Autodesk Inventor part; units mm, degrees
ref_plane "YZ Plane" through (0, 0, 0) normal (1, 0, 0) x (0, 1, 0)
ref_plane "XZ Plane" through (0, 0, 0) normal (0, 1, 0) x (-1, 0, 0)
ref_plane "XY Plane" through (0, 0, 0) normal (0, 0, 1) x (1, 0, 0)
sketch "Эскиз1" plane through (0, 0, 0) normal (0, 0, 1) x (1, 0, 0)
  line L0 (-4.6809, -0.7904) -> (-4.6809, 1.2096)
  line L1 (-4.6809, -13.7904) -> (-4.6809, -11.7904)
  line L2 (-4.6809, 1.2096) -> (-9.1809, 1.2096)
  line L3 (-10.1809, 0.2096) -> (-10.1809, -12.7904)
  line L4 (-9.1809, -13.7904) -> (-4.6809, -13.7904)
  arc A0 (-10.1809, -12.7904) -> (-9.1809, -13.7904) centre (-9.1809, -12.7904) ccw
  arc A1 (-9.1809, 1.2096) -> (-10.1809, 0.2096) centre (-9.1809, 0.2096) ccw
  line L5 (22.8191, -1.7904) -> (22.8191, -10.7904)
  line L6 (21.8191, -11.7904) -> (-4.6809, -11.7904)
  line L7 (-4.6809, -0.7904) -> (21.8191, -0.7904)
  arc A2 (22.8191, -1.7904) -> (21.8191, -0.7904) centre (21.8191, -1.7904) ccw
  arc A3 (21.8191, -11.7904) -> (22.8191, -10.7904) centre (21.8191, -10.7904) ccw
  arc A4 (-0.4309, -4.5404) -> (-0.4309, -8.0404) centre (-0.4309, -6.2904) ccw
  arc A5 (1.5691, -8.0404) -> (1.5691, -4.5404) centre (1.5691, -6.2904) ccw
  line L8 (-0.4309, -4.5404) -> (1.5691, -4.5404)
  line L9 (-0.4309, -8.0404) -> (1.5691, -8.0404)
  circle A6 centre (18.0691, -6.2904) radius 1.75
  point P0 (0, 0)
  point P1 (-10.1809, 1.2096)
  point P2 (-10.1809, -13.7904)
  point P3 (22.8191, -0.7904)
  point P4 (22.8191, -11.7904)
extrude "Выдавливание2" add sketch "Эскиз1" along normal blind 2
properties part number "Крепеж"
Here's how the part is built. I have some questions about the finished solid (model axes, mm). A direction names the side the tool comes from. Coordinates: 2 decimals unless noted, no trailing zeros. Order: outer loops, then holes, each group sorted by start corner. A loop starts at its lowest first (then second) coordinate and runs counter-clockwise, first axis right, second up.
Item 1: Which directions (+Z, -Z, +X, -X, +Y, -Y) give clear straight access to the entire face, cutting with the end or side of a thin tool? Please do faces 1 (the face through (6, -6, 0)), 2 (the face through (9, -11.79, 1)), 3 (the face through (-4.681, 0, 1)), 4 (the face through (1, -8.04, 1)), 5 (the face through (-9.88, -13.505, 0.986)).
Response values:
face 1: -Z, +X, -X, +Y, -Y
face 2: +Z, -Z, +X, -Y
face 3: +Z, -Z, +X, +Y
face 4: +Z, -Z
face 5: +Z, -Z, -X, -Y
Item 2: I'm going to push flat-ended pins straight in: pin 1 Ø1 at (y, z) = (0.5, 1.5) entering from +X; pin 2 Ø0.6 at (x, z) = (1, 1) entering from +Y; pin 3 Ø2 at (x, y) = (18.07, -6.29) entering from -Z; pin 4 Ø1 at (x, z) = (10, 1.5) entering from -Y. Where does each tip first touch, or does it pass through?
Response values:
pin 1: stops at x = -4.68
pin 2: stops at y = -0.79
pin 3: passes through
pin 4: stops at y = -11.79
Item 3: If we section it at C-C, the plane x = 8: List the corners of the cut face in (y, z) for me, then the cut area to 3 significant figures.
Response values:
outline: (-11.79, 0) - (-0.79, 0) - (-0.79, 2) - (-11.79, 2) - close
area: 22.0 mm2
Item 4: If we section it at B-B, the plane z = 1.25: List the corners of the cut face in (x, y) for me.
Response values:
outline: (-10.18, -12.79) arc R1 ccw to (-9.18, -13.79) - (-4.68, -13.79) - (-4.68, -11.79) - (21.82, -11.79) arc R1 ccw to (22.82, -10.79) - (22.82, -1.79) arc R1 ccw to (21.82, -0.79) - (-4.68, -0.79) - (-4.68, 1.21) - (-9.18, 1.21) arc R1 ccw to (-10.18, 0.21) - close; hole (-0.43, -8.04) - (1.57, -8.04) arc R1.75 ccw to (1.57, -4.54) - (-0.43, -4.54) arc R1.75 ccw to start; hole circle Ø3.5 at (18.07, -6.29)
Item 5: If we section it at A-A, the plane y = -7: List the corners of the cut face in (x, z) for me.
Response values:
outline: (-10.18, 0) - (-2.03, 0) - (-2.03, 2) - (-10.18, 2) - close; (3.17, 0) - (16.47, 0) - (16.47, 2) - (3.17, 2) - close; (19.67, 0) - (22.82, 0) - (22.82, 2) - (19.67, 2) - close
Item 6: Thinking about a two-plate mould opening in Y: for faces 6 (the face through (1, -4.54, 1)), 7 (the face through (-4.681, -13, 1)), 8 (the face through (-7, 1.21, 1)), which applies, pulls with the +Y half, pulls with the -Y half, needs draft (parallel to the pull), parting line crosses it, or undercut?
Response values:
face 6: undercut
face 7: needs draft
face 8: pulls with the +Y half
Item 7: I need wall thicknesses on probe 1 along X at (y, z) = (-7.5, 1.25); probe 2 along X at (y, z) = (-5.5, 0.5); probe 3 along Y at (x, z) = (11, 0.5). Which ranges of each line are inside material? Lowest first, please.
Response values:
probe 1: x = -10.18 to -1.7, 2.83 to 16.8, 19.33 to 22.82
probe 2: x = -10.18 to -1.99, 3.13 to 16.51, 19.63 to 22.82
probe 3: y = -11.79 to -0.79
